Read the model definition and answer for the solid it produces. Units are mm, in the model's axes. A direction names the side the tool comes from. Coordinates: 2 decimals unless noted, no trailing zeros. Order: outer loops, then holes, each group sorted by start corner. A loop starts at its lowest first (then second) coordinate and runs counter-clockwise, first axis right, second up.
```python
from build123d import *

# Parameters (mm, degrees)
SKETCH_W     = 1050
SKETCH_H     = 1050
PAD_DEPTH    = 1000
CHAMFER_SIZE = 200


with BuildPart() as chamfer_body:
    # Sketch → Pad (new body)
    with BuildSketch(Plane.XY):
        Rectangle(SKETCH_W, SKETCH_H)
    extrude(amount=PAD_DEPTH)

    # Chamfer
    chamfer_edges = [chamfer_body.edges().sort_by_distance(p)[0] for p in [
        (0, 525, 1000),
        (0, -525, 1000),
    ]]
    chamfer(chamfer_edges, length=CHAMFER_SIZE)


with BuildPart() as fusion:
    # Sweep: sweep along a path in Sketch001
    with BuildLine(Plane.XY) as sweep_path:
        Line((525, -525), (525, 525))
        Line((525, 525), (-525, 525))
        Line((-525, 525), (-525, -525))
        Line((-525, -525), (525, -525))
    # AngleSteel → Sweep (sweep)
    with BuildSketch(Plane(origin=(539.3963419701, 0, 14.3963419701), x_dir=(1, 0, 0), z_dir=(0, 1, 0))):
        with BuildLine():
            Line((-14.3963419701, 14.3963419701), (-14.3963419701, -35.6036580299))
            Line((-14.3963419701, -35.6036580299), (-12.8963419701, -35.6036580299))
            ThreePointArc((-12.8963419701, -35.6036580299), (-9.7143614548, -34.2856385452), (-8.3963419701, -31.1036580299))
            Line((-8.3963419701, -31.1036580299), (-8.3963419701, 1.8963419701))
            ThreePointArc((-8.3963419701, 1.8963419701), (-6.4925360478, 6.4925360478), (-1.8963419701, 8.3963419701))
            Line((-1.8963419701, 8.3963419701), (31.1036580299, 8.3963419701))
            ThreePointArc((31.1036580299, 8.3963419701), (34.2856385452, 9.7143614548), (35.6036580299, 12.8963419701))
            Line((35.6036580299, 12.8963419701), (35.6036580299, 14.3963419701))
            Line((35.6036580299, 14.3963419701), (-14.3963419701, 14.3963419701))
        make_face()
    sweep(path=sweep_path.line, is_frenet=True, transition=Transition.RIGHT)

    # Fusion: union Chamfer body
    add(chamfer_body.part)


with BuildPart() as fusion_1:
    # Fusion placement: moved
    add(fusion.part.moved(Location((0, 0, 186.5))))


solid = fusion_1.part
```
1) Which of the six approach directions +Z, -Z, +X, -X, +Y, -Y give full straight-line access (tool end or side, diameter ignored) to faces 1 (the flat face through (-7, -525, 606)), 2 (the flat face through (-531, -7, 216)), 3 (the flat face through (525, -7, 705))?
A:
face 1: +Z, +X, -X, -Y
face 2: +Z, -X, +Y, -Y
face 3: +Z, +X, +Y, -Y
2) A cutting plane is placed at A-A, the plane x = -445. Determine the outline of the cut face in (y, z).
A:
outline: (-575, 186.5) - (575, 186.5) - (575, 188) arc R4.5 ccw to (570.5, 192.5) - (537.5, 192.5) arc R6.5 cw to (531, 199) - (531, 232) arc R4.5 ccw to (526.5, 236.5) - (525, 236.5) - (525, 986.5) - (325, 1186.5) - (-325, 1186.5) - (-525, 986.5) - (-525, 236.5) - (-526.5, 236.5) arc R4.5 ccw to (-531, 232) - (-531, 199) arc R6.5 cw to (-537.5, 192.5) - (-570.5, 192.5) arc R4.5 ccw to (-575, 188) - close
3) A cutting plane is placed at B-B, the plane y = 418. Determine the outline of the cut face in (x, z), and give its area (3 significant figures).
A:
outline: (-575, 186.5) - (575, 186.5) - (575, 188) arc R4.5 ccw to (570.5, 192.5) - (537.5, 192.5) arc R6.5 cw to (531, 199) - (531, 232) arc R4.5 ccw to (526.5, 236.5) - (525, 236.5) - (525, 1093.5) - (-525, 1093.5) - (-525, 236.5) - (-526.5, 236.5) arc R4.5 ccw to (-531, 232) - (-531, 199) arc R6.5 cw to (-537.5, 192.5) - (-570.5, 192.5) arc R4.5 ccw to (-575, 188) - close
area: 953,000 mm2
4) A cutting plane is placed at D-D, the plane y = 181. Determine the outline of the cut face in (x, z), and give its area (3 significant figures).
A:
outline: (-575, 186.5) - (575, 186.5) - (575, 188) arc R4.5 ccw to (570.5, 192.5) - (537.5, 192.5) arc R6.5 cw to (531, 199) - (531, 232) arc R4.5 ccw to (526.5, 236.5) - (525, 236.5) - (525, 1186.5) - (-525, 1186.5) - (-525, 236.5) - (-526.5, 236.5) arc R4.5 ccw to (-531, 232) - (-531, 199) arc R6.5 cw to (-537.5, 192.5) - (-570.5, 192.5) arc R4.5 ccw to (-575, 188) - close
area: 1,050,000 mm2
5) Flat-ended cylindrical pins translate along their axes: pin 1 Ø6 at (y, z) = (-179, 443) entering from +X; pin 2 Ø1.5 at (x, z) = (-331, 824.5) entering from +Y; pin 3 Ø4 at (x, z) = (388, 669.5) entering from -Y. Find the tip coordinate at first contact, or state that the pin passes through.
A:
pin 1: stops at x = 525
pin 2: stops at y = 525
pin 3: stops at y = -525
6) A cutting plane is placed at C-C, the plane z = 1065. Determine the outline of the cut face in (x, y).
A:
outline: (-525, -446.5) - (525, -446.5) - (525, 446.5) - (-525, 446.5) - close
7) Straight lines are drawn through the part: line 1 (X direction, y = -25, z = 1010); line 2 (Z direction, x = -526, y = 314). For each, find the intervals that lie inside material, in ascending order.
A:
line 1: x = -525 to 525
line 2: z = 186.5 to 236.5
